from build123d import *

# Parameters (mm, degrees)
SKETCH1_W           = 10
SKETCH1_H           = 10
BOSS_EXTRUDE1_DEPTH = 1.5
SKETCH2_W           = 4
SKETCH2_H           = 4
BOSS_EXTRUDE2_DEPTH = 1.5
CUT_EXTRUDE1_DEPTH  = 1.5
CIRPATTERN1_COUNT   = 4


with BuildPart() as part:
    # Sketch1 → Boss-Extrude1 (new body)
    with BuildSketch(Plane(origin=(0, 0, 0), x_dir=(1, 0, 0), z_dir=(0, 1, 0))):
        Rectangle(SKETCH1_W, SKETCH1_H)
    extrude(amount=BOSS_EXTRUDE1_DEPTH)

    # Sketch2 → Boss-Extrude2 (add)
    with BuildSketch(Plane(origin=(0, 1.5, 0), x_dir=(1, 0, 0), z_dir=(0, 1, 0))):
        Rectangle(SKETCH2_W, SKETCH2_H)
    extrude(amount=BOSS_EXTRUDE2_DEPTH)

    # Sketch3 → Cut-Extrude1 (cut)
    with BuildSketch(Plane(origin=(0, 1.5, 0), x_dir=(1, 0, 0), z_dir=(0, 1, 0))):
        Polygon((-5, 2), (-2, 5), (-5, 5), align=None)
    cut_extrude1 = extrude(amount=-CUT_EXTRUDE1_DEPTH, mode=Mode.SUBTRACT)

    # CirPattern1: Cut-Extrude1 ×4 about axis
    cirpattern1_axis = Axis((0, 0, 0), (0, 1, 0))
    for i in range(1, CIRPATTERN1_COUNT):
        add(cut_extrude1.rotate(cirpattern1_axis, i * 360 / CIRPATTERN1_COUNT), mode=Mode.SUBTRACT)


solid = part.part
Part model, mm, in its own coordinate system. A direction names the side the tool comes from. Coordinates: 2 decimals unless noted, no trailing zeros. Loops run counter-clockwise (first coordinate to the right, second up) from the corner with the lowest first, then second, coordinate; pieces in that order, holes last. Notation, with made-up numbers: (71, 5) -> (130, 5) arc R19 cw to (130, 12) -> close; hole circle Ø5 at (-9, 78.5). An arc over 180 degrees is marked (long way). Use a Markdown table: item, result. Add a question column.
Item 1: Band-saw the part on C-C on z = -2.5. Write the cut outline in (x, y), plus the area to 3 significant figures.
Item 2: Band-saw the part on B-B on x = -1. Write the cut outline in (y, z), plus the area to 3 significant figures.
Item 3: Which spindle directions (+Z, -Z, +X, -X, +Y, -Y) get a long thin tool onto all of the face, cutting with end or side? Do faces 1 (the flat face through (0, 2, -2)), 2 (the flat face through (0, 2, 2)), 3 (the flat face through (-2, 2, 0)), 4 (the flat face through (2, 2, 0)). Say none if no direction does.
Item 4: Probe probe 1 along Z at (x, y) = (1.25, 2.5); probe 2 along Y at (x, z) = (-4.25, 2.5). List the from-to ranges inside material, lowest first.
Item 5: Flat gauge pins, fed straight in: P1, Ø0.8, axis at y = 2.5, z = -0.5, coming from the +X side; P2, Ø1.2, axis at y = 2.5, z = -0.5, coming from the -X side; P3, Ø0.8, axis at x = 0, y = 2.5, coming from the +Z side. Where does each tip first touch, or does it go through?
Item 6: Band-saw the part on D-D on x = -4. Write the cut outline in (y, z).
Item 7: Band-saw the part on A-A on y = 0.9. Write the cut outline in (x, z), plus the area to 3 significant figures.
Geometry says:
| question | item | result |
|---|---|---|
| 1 | outline | (-4.5, 0) -> (4.5, 0) -> (4.5, 1.5) -> (-4.5, 1.5) -> close |
| 1 | area | 13.5 mm² |
| 2 | outline | (0, -5) -> (1.5, -5) -> (1.5, -2) -> (3, -2) -> (3, 2) -> (1.5, 2) -> (1.5, 5) -> (0, 5) -> close |
| 2 | area | 21.0 mm² |
| 3 | face 1 | -Z, +X, -X, +Y |
| 3 | face 2 | +Z, +X, -X, +Y |
| 3 | face 3 | +Z, -Z, -X, +Y |
| 3 | face 4 | +Z, -Z, +X, +Y |
| 4 | probe 1 | -2 to 2 |
| 4 | probe 2 | 0 to 1.5 |
| 5 | P1 | x = 2 |
| 5 | P2 | x = -2 |
| 5 | P3 | z = 2 |
| 6 | outline | (0, -3) -> (1.5, -3) -> (1.5, 3) -> (0, 3) -> close |
| 7 | outline | (-5, -2) -> (-2, -5) -> (2, -5) -> (5, -2) -> (5, 2) -> (2, 5) -> (-2, 5) -> (-5, 2) -> close |
| 7 | area | 82.0 mm² |
